Can you work these out from the model? Positions are in its coordinate system, mm. Face numbers are marked on the shaded views. Coordinates: 2 decimals unless noted, no trailing zeros. Order: outer loops, then holes, each group sorted by start corner. A loop starts at its lowest first (then second) coordinate and runs counter-clockwise, first axis right, second up. Notation, with made-up numbers: (10.25, 77.5) -> (20.25, 77.5) arc R7 cw to (20.25, 88.5) -> close; hole circle Ø9 at (-22, 54). An arc over 180 degrees is marked (long way). Answer as a JSON object with one key per item and string values. Group by question number.
(1) If we mould it in two halves opening along Z, with no side actions, what happens to the marked faces 1 and 2? For each: pulls with the +Z half, pulls with the -Z half, needs draft (parallel to the pull), parting line crosses it, or undercut.
(2) I want a section at B-B, the plane x = 0. List the corners of the cut face in (y, z) for me.
(3) I need wall thicknesses on line 1 (Z direction, x = 0, y = 4.75); line 2 (X direction, y = 3.25, z = -23.5); line 3 (Z direction, x = -38, y = 4). Which ranges of each line are inside material? Lowest first, please.
(4) I want a section at A-A, the plane z = 0. List the corners of the cut face in (x, y) for me, plus the area to 3 significant figures.
(5) For pin 1 (1.5 mm diameter, centred on x = 21.5, y = 7, fed in from +Z); pin 2 (3.5 mm diameter, centred on x = -38.8, z = 22.4, fed in from +Y); pin 3 (2 mm diameter, centred on x = 9, y = 9, fed in from -Z); pin 4 (2 mm diameter, centred on x = -8.5, y = 5.5, fed in from +Z), each with a flat end and sliding along its axis, tell me the tip position at first contact or that it passes through.
(6) I want a section at D-D, the plane y = 5.5. List the corners of the cut face in (x, z) for me, plus the area to 3 significant figures.
(7) I want a section at C-C, the plane z = 22.4. List the corners of the cut face in (x, y) for me, plus the area to 3 significant figures.
from build123d import *

# Parameters (mm, degrees)
SKETCH1_R           = 50.8
BOSS_EXTRUDE1_DEPTH = 10
SKETCH2_R           = 38.1
SKETCH2_R_2         = 36.5
CUT_EXTRUDE1_DEPTH  = 2
SKETCH3_R           = 2
CUT_EXTRUDE2_DEPTH  = 14


with BuildPart() as part:
    # Sketch1 → Boss-Extrude1 (new body)
    with BuildSketch(Plane(origin=(0, 0, 0), x_dir=(1, 0, 0), z_dir=(0, 1, 0))):
        Circle(SKETCH1_R)
    extrude(amount=BOSS_EXTRUDE1_DEPTH)

    # Sketch2 → Cut-Extrude1 (cut)
    with BuildSketch(Plane.XZ):
        Circle(SKETCH2_R)
        Circle(SKETCH2_R_2, mode=Mode.SUBTRACT)
    extrude(amount=-CUT_EXTRUDE1_DEPTH, mode=Mode.SUBTRACT)

    # Sketch3 → Cut-Extrude2 (cut)
    with BuildSketch(Plane(origin=(0, 10, 0), x_dir=(1, 0, 0), z_dir=(0, 1, 0))):
        Circle(SKETCH3_R)
        with Locations((0, 44.8)):
            Circle(SKETCH3_R)
        with Locations((38.79793809, 22.4)):
            Circle(SKETCH3_R)
        with Locations((38.79793809, -22.4)):
            Circle(SKETCH3_R)
        with Locations((0, -44.8)):
            Circle(SKETCH3_R)
        with Locations((-38.79793809, -22.4)):
            Circle(SKETCH3_R)
        with Locations((-38.79793809, 22.4)):
            Circle(SKETCH3_R)
    extrude(amount=-CUT_EXTRUDE2_DEPTH, mode=Mode.SUBTRACT)


solid = part.part
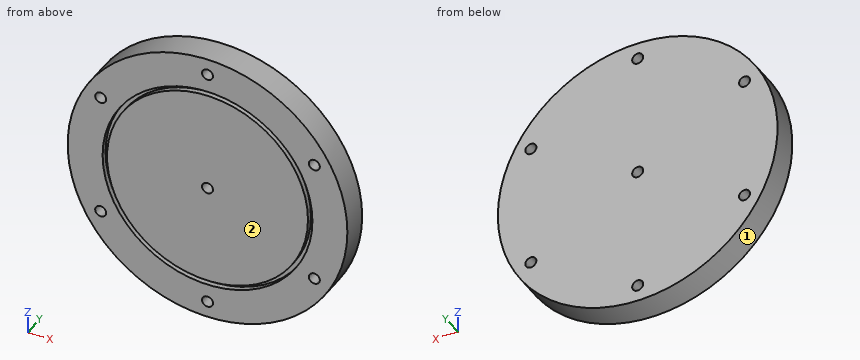
Computed values:
{
 "1": {"face 1": "parting line crosses it", "face 2": "needs draft"},
 "2": {"outline": "(0, -50.8) -> (10, -50.8) -> (10, -46.8) -> (0, -46.8) -> close; (0, -42.8) -> (10, -42.8) -> (10, -2) -> (0, -2) -> (0, -36.5) -> (2, -36.5) -> (2, -38.1) -> (0, -38.1) -> close; (0, 2) -> (10, 2) -> (10, 42.8) -> (0, 42.8) -> (0, 38.1) -> (2, 38.1) -> (2, 36.5) -> (0, 36.5) -> close; (0, 46.8) -> (10, 46.8) -> (10, 50.8) -> (0, 50.8) -> close"},
 "3": {"line 1": "z = -50.8 to -46.8, -42.8 to -2, 2 to 42.8, 46.8 to 50.8", "line 2": "x = -45.04 to -40.47, -37.13 to 37.13, 40.47 to 45.04", "line 3": "z = -33.71 to -24.23, -20.57 to 20.57, 24.23 to 33.71"},
 "4": {"outline": "(-50.8, 0) -> (-38.1, 0) -> (-38.1, 2) -> (-36.5, 2) -> (-36.5, 0) -> (-2, 0) -> (-2, 10) -> (-50.8, 10) -> close; (2, 0) -> (36.5, 0) -> (36.5, 2) -> (38.1, 2) -> (38.1, 0) -> (50.8, 0) -> (50.8, 10) -> (2, 10) -> close", "area": "970 mm2"},
 "5": {"pin 1": "stops at z = 46.37", "pin 2": "passes through", "pin 3": "stops at z = -50.17", "pin 4": "stops at z = 50.24"},
 "6": {"outline": "circle Ø101.6 at (0, 0); hole circle Ø4 at (-38.8, -22.4); hole circle Ø4 at (-38.8, 22.4); hole circle Ø4 at (0, -44.8); hole circle Ø4 at (0, 0); hole circle Ø4 at (0, 44.8); hole circle Ø4 at (38.8, -22.4); hole circle Ø4 at (38.8, 22.4)", "area": "8,020 mm2"},
 "7": {"outline": "(-45.59, 0) -> (-40.8, 0) -> (-40.8, 10) -> (-45.59, 10) -> close; (-36.8, 0) -> (-30.82, 0) -> (-30.82, 2) -> (-28.82, 2) -> (-28.82, 0) -> (28.82, 0) -> (28.82, 2) -> (30.82, 2) -> (30.82, 0) -> (36.8, 0) -> (36.8, 10) -> (-36.8, 10) -> close; (40.8, 0) -> (45.59, 0) -> (45.59, 10) -> (40.8, 10) -> close", "area": "824 mm2"}
}
